Design review of the part built by this model. Coordinates are the model's own, in mm. Face numbers are marked on the shaded views. A direction names the side the tool comes from. Coordinates: 2 decimals unless noted, no trailing zeros. Write each loop counter-clockwise with the first axis right and the second up, starting at its lowest first coordinate (ties: lowest second). Pieces come first, ordered by that corner, then holes. Notation, with made-up numbers: (29, 80) - (71, 80) arc R31 ccw to (71, 114) - close; hole circle Ø9 at (80.5, 58). An arc over 180 degrees is marked (long way). Use a Markdown table: item, result.
from build123d import *

# Parameters (mm, degrees)
F0_W     = 19.05
F0_H     = 19.05
F1_DEPTH = 6.223
F2_W     = 19.05
F2_H     = 19.05
F2_R     = 6.985
F3_DEPTH = 2.54
F4_R     = 1.4732
F5_DEPTH = 3.684
F6_W     = 19.05
F6_H     = 19.05
F6_R     = 1.5875
F7_DEPTH = 0.508
F8_R     = 1.5875
F9_DEPTH = 1.016


with BuildPart() as f1:
    # F0 (on Top) → F1 (new body)
    with BuildSketch(Plane.XY):
        Rectangle(F0_W, F0_H)
    extrude(amount=F1_DEPTH)

    # F2 (on face) → F3 (cut)
    with BuildSketch(Plane.XY.offset(6.223)):
        Rectangle(F2_W, F2_H)
        Circle(F2_R, mode=Mode.SUBTRACT)
    extrude(amount=-F3_DEPTH, mode=Mode.SUBTRACT)

    # F4 (on face) → F5 (cut, through all)
    with BuildSketch(Plane.XY.offset(3.683)):
        with Locations((-7.239, 7.239)):
            Circle(F4_R)
        with Locations((-7.239, -6.731)):
            Circle(F4_R)
        with Locations((6.731, 7.239)):
            Circle(F4_R)
        with Locations((6.731, -6.731)):
            Circle(F4_R)
    extrude(amount=-F5_DEPTH, mode=Mode.SUBTRACT)

    # F6 (on face) → F7 (cut)
    with BuildSketch(Plane(origin=(0, 0, 0), x_dir=(1, 0, 0), z_dir=(0, 0, -1))):
        Rectangle(F6_W, F6_H)
        Circle(F6_R, mode=Mode.SUBTRACT)
    extrude(amount=-F7_DEPTH, mode=Mode.SUBTRACT)

    # F8 (on face) → F9 (cut)
    with BuildSketch(Plane(origin=(0, 0, 0.508), x_dir=(1, 0, 0), z_dir=(0, 0, -1))):
        with BuildLine():
            ThreePointArc((-2.1236319767, -1.0912474455), (-1.8017283129, -0.5872901809), (-1.6891, 0))
            ThreePointArc((-1.6891, 0), (-1.8017283129, 0.5872901809), (-2.1236319767, 1.0912474455))
            ThreePointArc((-2.1236319767, 1.0912474455), (-2.3876, 0), (-2.1236319767, -1.0912474455))
        make_face()
        with BuildLine():
            ThreePointArc((-2.1236319767, 1.0912474455), (-1.8017283129, 0.5872901809), (-1.6891, 0))
            ThreePointArc((-1.6891, 0), (-1.8017283129, -0.5872901809), (-2.1236319767, -1.0912474455))
            ThreePointArc((-2.1236319767, -1.0912474455), (0.5613599791, -2.320669889), (2.3876, 0))
            ThreePointArc((2.3876, 0), (0.5613599791, 2.320669889), (-2.1236319767, 1.0912474455))
        make_face()
        Circle(F8_R, mode=Mode.SUBTRACT)
        with BuildLine():
            ThreePointArc((-2.1236319767, -1.0912474455), (-2.3876, 0), (-2.1236319767, 1.0912474455))
            ThreePointArc((-2.1236319767, 1.0912474455), (-4.8641, 0), (-2.1236319767, -1.0912474455))
        make_face()
    extrude(amount=-F9_DEPTH, mode=Mode.SUBTRACT)


solid = f1.part
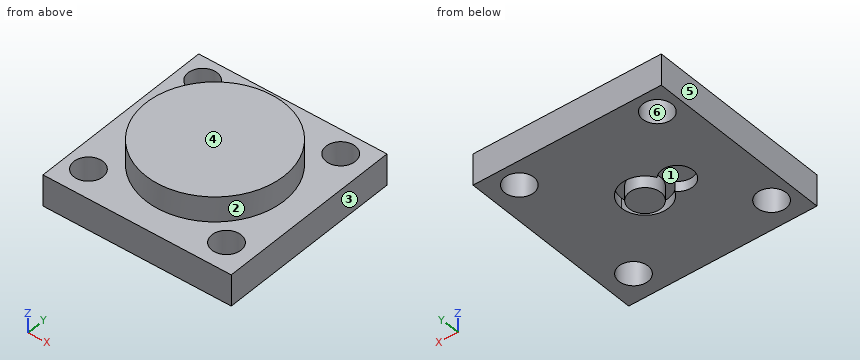
(1) Draft analysis for pull direction X (two halves, no side actions). For the marked faces 4, 5 and 6, state which applies: +X half, -X half, draft (parallel to the pull), parting line (faces both ways), or undercut.
Determined:
| item | result |
|---|---|
| face 4 | draft |
| face 5 | -X half |
| face 6 | undercut |
(2) Machinability: for the marked faces 1, 2 and 3, which of the approach directions +Z, -Z, +X, -X, +Y, -Y give a long, thin tool a straight path to every point of the face, cutting with its end or side? Answer none if there is none.
Determined:
| item | result |
|---|---|
| face 1 | -Z |
| face 2 | +Z |
| face 3 | +Z, -Z, +X, +Y, -Y |
(3) For pin 1 (4.5 mm diameter, centred on x = -7.239, y = -6.731, fed in from -Z); pin 2 (1.8 mm diameter, centred on x = 6.731, y = 7.239, fed in from +Z); pin 3 (1 mm diameter, centred on y = -1.5, z = 5, fed in from -X), all flat-tipped, find the tip position at first contact; note any pin that passes through.
Determined:
| item | result |
|---|---|
| pin 1 | z = 0.51 |
| pin 2 | through |
| pin 3 | x = -6.91 |
(4) Take a section at B-B on z = 2.5. Write out the cut boundary in (x, y) (3 decimals), and give its area (3 significant figures).
Determined:
| item | result |
|---|---|
| outline | (-9.525, -9.525) - (9.525, -9.525) - (9.525, 9.525) - (-9.525, 9.525) - close; hole circle Ø2.946 at (-7.239, -6.731); hole circle Ø2.946 at (-7.239, 7.239); hole circle Ø2.946 at (6.731, -6.731); hole circle Ø2.946 at (6.731, 7.239) |
| area | 336 mm2 |
(5) For L1, parallel to X at y = 7.25, z = 3 (3 decimals); L2, parallel to Z at x = -7.25, y = 2; L3, parallel to Z at x = -6, y = -1.75, list the stretches that pass through material, from the lowest coordinate up. Write a range as from..to.
Determined:
| item | result |
|---|---|
| L1 | -9.525..-8.712, -5.766..5.258, 8.204..9.525 |
| L2 | 0.51..3.68 |
| L3 | 0.51..6.22 |
(6) Take a section at A-A on x = 0. Write out the cut boundary in (y, z) (1 decimal), and give its area (3 significant figures).
Determined:
| item | result |
|---|---|
| outline | (-9.5, 0.5) - (-2.4, 0.5) - (-2.4, 1.5) - (-1.6, 1.5) - (-1.6, 0) - (1.6, 0) - (1.6, 1.5) - (2.4, 1.5) - (2.4, 0.5) - (9.5, 0.5) - (9.5, 3.7) - (7, 3.7) - (7, 6.2) - (-7, 6.2) - (-7, 3.7) - (-9.5, 3.7) - close |
| area | 96.0 mm2 |
(7) Take a section at C-C on y = 5.5. Write out the cut boundary in (x, z) (3 decimals).
Determined:
| item | result |
|---|---|
| outline | (-9.525, 0.508) - (9.525, 0.508) - (9.525, 3.683) - (4.306, 3.683) - (4.306, 6.223) - (-4.306, 6.223) - (-4.306, 3.683) - (-9.525, 3.683) - close |
(8) Take a section at D-D on z = 4.5. Write out the cut boundary in (x, y) (3 decimals).
Determined:
| item | result |
|---|---|
| outline | circle Ø13.97 at (0, 0) |
